```python
from build123d import *

# Parameters (mm, degrees)
F0_R     = 1.905
F1_DEPTH = 2.032
F2_DEPTH = 2.54
F3_R     = 1.016


# Not quite as in the source:
# - a feature names something its author has since deleted; it is built from what else it names


with BuildPart() as f1:
    # F0 (on Top) → F1 (new body)
    with BuildSketch(Plane.XY):
        with BuildLine():
            Line((6.35, 4.6835285843), (6.35, 7.0710607408))
            ThreePointArc((6.35, 7.0710607408), (3.4516559454, 8.1852117072), (0.3466541063, 8.1588637779))
            ThreePointArc((0.3466541063, 8.1588637779), (-4.4614598428, 5.2775997073), (-6.35, 1.93e-08))
            ThreePointArc((-6.35, 1.93e-08), (-4.4614598575, -5.2775996893), (0.3466540985, -8.1588637764))
            ThreePointArc((0.3466540985, -8.1588637764), (3.4516559415, -8.1852117079), (6.35, -7.0710607408))
            Line((6.35, -7.0710607408), (6.35, -4.6835285843))
            ThreePointArc((6.35, -4.6835285843), (-4.445, 0), (6.35, 4.6835285843))
        make_face()
        with BuildLine():
            ThreePointArc((10.287, 0), (9.2364071953, 4.0465994675), (6.35, 7.0710607408))
            Line((6.35, 7.0710607408), (6.35, 4.6835285843))
            ThreePointArc((6.35, 4.6835285843), (7.8521099675, 2.5526684078), (8.382, 0))
            ThreePointArc((8.382, 0), (7.8521099675, -2.5526684078), (6.35, -4.6835285843))
            Line((6.35, -4.6835285843), (6.35, -7.0710607408))
            ThreePointArc((6.35, -7.0710607408), (9.2364071953, -4.0465994675), (10.287, 0))
        make_face()
        with BuildLine():
            Line((-1.778, 9.9027430543), (-1.778, 12.7))
            Line((-1.778, 12.7), (-6.35, 12.7))
            Line((-6.35, 12.7), (-6.35, 1.93e-08))
            ThreePointArc((-6.35, 1.93e-08), (-4.4614598428, 5.2775997073), (0.3466541063, 8.1588637779))
            ThreePointArc((0.3466541063, 8.1588637779), (-1.1280365683, 8.528400484), (-1.778, 9.9027430543))
        make_face()
        with BuildLine():
            Line((6.35, 7.0710607408), (6.35, 12.7))
            Line((6.35, 12.7), (1.778, 12.7))
            Line((1.778, 12.7), (1.778, 9.9027430543))
            ThreePointArc((1.778, 9.9027430543), (1.3743425703, 8.774706486), (0.3466541063, 8.1588637779))
            ThreePointArc((0.3466541063, 8.1588637779), (3.4516559454, 8.1852117072), (6.35, 7.0710607408))
        make_face()
        with BuildLine():
            Line((6.35, -12.7), (6.35, -7.0710607408))
            ThreePointArc((6.35, -7.0710607408), (3.4516559415, -8.1852117079), (0.3466540985, -8.1588637764))
            ThreePointArc((0.3466540985, -8.1588637764), (1.3743425678, -8.7747064829), (1.778, -9.9027430543))
            Line((1.778, -9.9027430543), (1.778, -12.7))
            Line((1.778, -12.7), (6.35, -12.7))
        make_face()
        with BuildLine():
            ThreePointArc((0.3466540985, -8.1588637764), (-4.4614598575, -5.2775996893), (-6.35, 1.93e-08))
            Line((-6.35, 1.93e-08), (-6.35, -12.7))
            Line((-6.35, -12.7), (-1.778, -12.7))
            Line((-1.778, -12.7), (-1.778, -9.9027430543))
            ThreePointArc((-1.778, -9.9027430543), (-1.1280365714, -8.5284004866), (0.3466540985, -8.1588637764))
        make_face()
        with BuildLine():
            Line((6.35, -4.6835285843), (6.35, 4.6835285843))
            ThreePointArc((6.35, 4.6835285843), (-4.445, 0), (6.35, -4.6835285843))
        make_face()
        with Locations((1.9685, 0)):
            Circle(F0_R, mode=Mode.SUBTRACT)
        with BuildLine():
            ThreePointArc((8.382, 0), (7.8521099675, 2.5526684078), (6.35, 4.6835285843))
            Line((6.35, 4.6835285843), (6.35, -4.6835285843))
            ThreePointArc((6.35, -4.6835285843), (7.8521099675, -2.5526684078), (8.382, 0))
        make_face()
    extrude(amount=-F1_DEPTH)

    # F0 (on Top) → F2 (join)
    with BuildSketch(Plane.XY):
        with BuildLine():
            Line((6.35, 4.6835285843), (6.35, 7.0710607408))
            ThreePointArc((6.35, 7.0710607408), (3.4516559454, 8.1852117072), (0.3466541063, 8.1588637779))
            ThreePointArc((0.3466541063, 8.1588637779), (-4.4614598428, 5.2775997073), (-6.35, 1.93e-08))
            ThreePointArc((-6.35, 1.93e-08), (-4.4614598575, -5.2775996893), (0.3466540985, -8.1588637764))
            ThreePointArc((0.3466540985, -8.1588637764), (3.4516559415, -8.1852117079), (6.35, -7.0710607408))
            Line((6.35, -7.0710607408), (6.35, -4.6835285843))
            ThreePointArc((6.35, -4.6835285843), (-4.445, 0), (6.35, 4.6835285843))
        make_face()
        with BuildLine():
            ThreePointArc((10.287, 0), (9.2364071953, 4.0465994675), (6.35, 7.0710607408))
            Line((6.35, 7.0710607408), (6.35, 4.6835285843))
            ThreePointArc((6.35, 4.6835285843), (7.8521099675, 2.5526684078), (8.382, 0))
            ThreePointArc((8.382, 0), (7.8521099675, -2.5526684078), (6.35, -4.6835285843))
            Line((6.35, -4.6835285843), (6.35, -7.0710607408))
            ThreePointArc((6.35, -7.0710607408), (9.2364071953, -4.0465994675), (10.287, 0))
        make_face()
        with BuildLine():
            Line((6.35, 7.0710607408), (6.35, 12.7))
            Line((6.35, 12.7), (1.778, 12.7))
            Line((1.778, 12.7), (1.778, 9.9027430543))
            ThreePointArc((1.778, 9.9027430543), (1.3743425703, 8.774706486), (0.3466541063, 8.1588637779))
            ThreePointArc((0.3466541063, 8.1588637779), (3.4516559454, 8.1852117072), (6.35, 7.0710607408))
        make_face()
        with BuildLine():
            Line((-1.778, 9.9027430543), (-1.778, 12.7))
            Line((-1.778, 12.7), (-6.35, 12.7))
            Line((-6.35, 12.7), (-6.35, 1.93e-08))
            ThreePointArc((-6.35, 1.93e-08), (-4.4614598428, 5.2775997073), (0.3466541063, 8.1588637779))
            ThreePointArc((0.3466541063, 8.1588637779), (-1.1280365683, 8.528400484), (-1.778, 9.9027430543))
        make_face()
        with BuildLine():
            Line((6.35, -12.7), (6.35, -7.0710607408))
            ThreePointArc((6.35, -7.0710607408), (3.4516559415, -8.1852117079), (0.3466540985, -8.1588637764))
            ThreePointArc((0.3466540985, -8.1588637764), (1.3743425678, -8.7747064829), (1.778, -9.9027430543))
            Line((1.778, -9.9027430543), (1.778, -12.7))
            Line((1.778, -12.7), (6.35, -12.7))
        make_face()
        with BuildLine():
            ThreePointArc((0.3466540985, -8.1588637764), (-4.4614598575, -5.2775996893), (-6.35, 1.93e-08))
            Line((-6.35, 1.93e-08), (-6.35, -12.7))
            Line((-6.35, -12.7), (-1.778, -12.7))
            Line((-1.778, -12.7), (-1.778, -9.9027430543))
            ThreePointArc((-1.778, -9.9027430543), (-1.1280365714, -8.5284004866), (0.3466540985, -8.1588637764))
        make_face()
    extrude(amount=F2_DEPTH)

    # F3
    f3_edges = [f1.edges().sort_by_distance(p)[0] for p in [
        (-2.413, -4.683529, 2.54),
    ]]
    fillet(f3_edges, radius=F3_R)


solid = f1.part
```
Build history of the part. All positions in model axes, mm. Coordinates: 2 decimals unless noted, no trailing zeros. Write each loop counter-clockwise with the first axis right and the second up, starting at its lowest first coordinate (ties: lowest second). Pieces come first, ordered by that corner, then holes.
1. Pull direction X, two halves, no side cores. Call faces 1 (the flat face through (3, 2, 0)), 2 (the flat face through (-2, 0, -2.032)): released by +X, released by -X, zero draft, split by the parting line, or undercut.
Answer block:
face 1: undercut
face 2: zero draft
2. Drill centre lines: probe 1 along X at (y, z) = (11.75, 1.65); probe 2 along Z at (x, y) = (-3.5, -3.25); probe 3 along X at (y, z) = (0, 1.2) (3 decimals). Where is each one in solid material? Low to high.
Answer block:
probe 1: x = -6.35 to -1.78, 1.78 to 6.35
probe 2: z = -2.03 to 0
probe 3: x = -6.35 to -4.445, 8.382 to 10.287
3. Band-saw the part on C-C, the plane z = 0.8. Give the cut face in (x, y).
Answer block:
outline: (-6.35, -12.7) - (-1.78, -12.7) - (-1.78, -9.9) arc R1.78 cw to (1.78, -9.9) - (1.78, -12.7) - (6.35, -12.7) - (6.35, -7.07) arc R8.32 ccw to (6.35, 7.07) - (6.35, 12.7) - (1.78, 12.7) - (1.78, 9.9) arc R1.78 cw to (-1.78, 9.9) - (-1.78, 12.7) - (-6.35, 12.7) - close; hole circle Ø12.83 at (1.97, 0)
4. Drop flat-ended pins along their axis: pin 1 (0.8 mm diameter, centred on y = 8.5, z = 1, fed in from +X); pin 2 (2 mm diameter, centred on y = -10.5, z = 1.5, fed in from +X); pin 3 (3 mm diameter, centred on x = 4.5, y = -1.5, fed in from +Z); pin 4 (2.5 mm diameter, centred on x = 1.97, y = 0, fed in from -Z). Give the stop position or say it passes through.
Answer block:
pin 1: stops at x = 6.35
pin 2: stops at x = 6.35
pin 3: stops at z = 0
pin 4: passes through
5. Band-saw the part on B-B, the plane y = -8.75. Give the cut face in (x, z).
Answer block:
outline: (-6.35, -2.03) - (-1.35, -2.03) - (-1.35, 2.54) - (-6.35, 2.54) - close; (1.35, -2.03) - (6.35, -2.03) - (6.35, 2.54) - (1.35, 2.54) - close
